from build123d import *

# Parameters (mm, degrees)
SKETCH1_W                  = 170
SKETCH1_H                  = 20
BOSS_EXTRUDE1_DEPTH        = 130
SKETCH2_R                  = 30
SKETCH2_R_2                = 15
BOSS_EXTRUDE3_DEPTH        = 60
BOSS_EXTRUDE3_DEPTH_BACK   = 6
BOSS_EXTRUDE3_2_DEPTH      = 60
BOSS_EXTRUDE3_2_DEPTH_BACK = 6
SKETCH2_4_W                = 55
SKETCH2_4_H                = 55
BOSS_EXTRUDE4_DEPTH        = 6
BOSS_EXTRUDE4_DEPTH_BACK   = 6
SKETCH2_5_W                = 55
SKETCH2_5_H                = 55
SKETCH2_5_R                = 20
BOSS_EXTRUDE5_DEPTH        = 100
RIB10_REACH                = 192.076
SKETCH3_WALL_W             = 453.9773952
SKETCH3_WALL_H             = 15
SKETCH4_R                  = 13
CUT_EXTRUDE1_DEPTH         = 217.573313222


with BuildPart() as part:
    # Sketch1 → Boss-Extrude1 (new body)
    with BuildSketch(Plane.XY):
        Rectangle(SKETCH1_W, SKETCH1_H)
    extrude(amount=-BOSS_EXTRUDE1_DEPTH)



with BuildPart() as body_2:
    # Sketch2 → Boss-Extrude3 (new, two sides)
    with BuildSketch(Plane(origin=(0, 0, 0), x_dir=(1, 0, 0), z_dir=(0, 1, 0))) as boss_extrude3_sk:
        with Locations(Location((-118, 65, 0), (0, 0, 270))):
            Circle(SKETCH2_R)
        with Locations(Location((-118, 65, 0), (0, 0, 270))):
            Circle(SKETCH2_R_2, mode=Mode.SUBTRACT)
    extrude(amount=BOSS_EXTRUDE3_DEPTH)
    extrude(boss_extrude3_sk.sketch, amount=-BOSS_EXTRUDE3_DEPTH_BACK)


with BuildPart() as body_3:
    # Sketch2 → Boss-Extrude3 2 (new, two sides)
    with BuildSketch(Plane(origin=(0, 0, 0), x_dir=(1, 0, 0), z_dir=(0, 1, 0))) as boss_extrude3_2_sk:
        with Locations(Location((118, 65, 0), (0, 0, 270))):
            Circle(SKETCH2_R)
        with Locations(Location((118, 65, 0), (0, 0, 270))):
            Circle(SKETCH2_R_2, mode=Mode.SUBTRACT)
    extrude(amount=BOSS_EXTRUDE3_2_DEPTH)
    extrude(boss_extrude3_2_sk.sketch, amount=-BOSS_EXTRUDE3_2_DEPTH_BACK)


with BuildPart() as part_1:
    add(part.part)

    add(body_2.part)  # Boss-Extrude4 merges body 2

    add(body_3.part)  # Boss-Extrude4 merges body 3
    # Sketch2_4 → Boss-Extrude4 (add, two sides)
    with BuildSketch(Plane(origin=(0, 0, 0), x_dir=(1, 0, 0), z_dir=(0, 1, 0))) as boss_extrude4_sk:
        with BuildLine():
            Line((85, 130), (-85, 130))
            Line((-85, 130), (-85, 110))
            ThreePointArc((-85, 110), (-89.393398282, 99.393398282), (-100, 95))
            Line((-100, 95), (-118, 95))
            ThreePointArc((-118, 95), (-96.786796564, 86.213203436), (-88, 65))
            ThreePointArc((-88, 65), (-96.786796564, 43.786796564), (-118, 35))
            Line((-118, 35), (-100, 35))
            ThreePointArc((-100, 35), (-89.393398282, 30.606601718), (-85, 20))
            Line((-85, 20), (-85, 0))
            Line((-85, 0), (85, 0))
            Line((85, 0), (85, 20))
            ThreePointArc((85, 20), (89.393398282, 30.606601718), (100, 35))
            Line((100, 35), (118, 35))
            ThreePointArc((118, 35), (88, 65), (118, 95))
            Line((118, 95), (100, 95))
            ThreePointArc((100, 95), (89.393398282, 99.393398282), (85, 110))
            Line((85, 110), (85, 130))
        make_face()
        with Locations((0, 65)):
            Rectangle(SKETCH2_4_W, SKETCH2_4_H, mode=Mode.SUBTRACT)
    extrude(amount=BOSS_EXTRUDE4_DEPTH)
    extrude(boss_extrude4_sk.sketch, amount=-BOSS_EXTRUDE4_DEPTH_BACK)

    # Sketch2_5 → Boss-Extrude5 (add)
    with BuildSketch(Plane(origin=(0, 0, 0), x_dir=(1, 0, 0), z_dir=(0, 1, 0))):
        with Locations((0, 65)):
            Rectangle(SKETCH2_5_W, SKETCH2_5_H)
        with Locations(Location((0, 65, 0), (0, 0, 270))):
            Circle(SKETCH2_5_R, mode=Mode.SUBTRACT)
    extrude(amount=BOSS_EXTRUDE5_DEPTH)

    # Sketch3 wall → Rib10 (add, up to next)
    with BuildSketch(Plane(origin=(-58.860010645, 77.5, -65), x_dir=(-0.873236351537, -0.487296905752, 0), z_dir=(0.487296905752, -0.873236351537, 0)), mode=Mode.PRIVATE) as rib10_sk1:
        Rectangle(SKETCH3_WALL_W, SKETCH3_WALL_H)
    rib10_tool1 = extrude(rib10_sk1.sketch, amount=RIB10_REACH, mode=Mode.PRIVATE) - part_1.part
    rib10 = rib10_tool1.solids().sort_by_distance((-58.860010645, 77.5, -65))[0]
    add(rib10)

    # Mirror1: Rib10 across plane
    add(rib10.mirror(Plane(origin=(0, 0, 0), x_dir=(0, 0, 1), z_dir=(1, 0, 0))))

    # Sketch4 → Cut-Extrude1 (cut, through all)
    with BuildSketch(Plane(origin=(0, 10, 0), x_dir=(1, 0, 0), z_dir=(0, 1, 0))):
        with Locations(Location((-63, 108, 0), (0, 0, 270))):
            Circle(SKETCH4_R)
        with Locations(Location((63, 108, 0), (0, 0, 270))):
            Circle(SKETCH4_R)
        with Locations(Location((-63, 22, 0), (0, 0, 270))):
            Circle(SKETCH4_R)
        with Locations(Location((63, 22, 0), (0, 0, 270))):
            Circle(SKETCH4_R)
    extrude(amount=-CUT_EXTRUDE1_DEPTH, mode=Mode.SUBTRACT)


solid = part_1.part
Can you work these out from the model? Positions are in its coordinate system, mm. A direction names the side the tool comes from. Give positions to 0.01 mm unless a question says otherwise; leave off trailing zeros. Loops run counter-clockwise (first coordinate to the right, second up) from the corner with the lowest first, then second, coordinate; pieces in that order, holes last. Notation, with made-up numbers: (63.5, -34.75) - (73.5, -34.75) arc R25 cw to (73.5, -9.75) - close; hole circle Ø1 at (-6, -21.75). An arc over 180 degrees is marked (long way). Answer as a JSON object with one key per item and string values.
Q1. Imagine slicing it at A-A on z = -65. Write out the boundary of the cut face in (x, y).
Geometry says:
{"outline": "(-148, -6) - (-133, -6) - (-133, 60) - (-148, 60) - close; (-103, -6) - (-85, -6) - (-85, -10) - (85, -10) - (85, -6) - (103, -6) - (103, 60) - (90.22, 60) - (27.5, 95) - (27.5, 100) - (20, 100) - (20, 10) - (-20, 10) - (-20, 100) - (-27.5, 100) - (-27.5, 95) - (-90.22, 60) - (-103, 60) - close; (133, -6) - (148, -6) - (148, 60) - (133, 60) - close"}
Q2. Imagine slicing it at B-B on y = 3. Write out the boundary of the cut face in (x, z), plus the area to 3 significant figures.
Geometry says:
{"outline": "(-118, -95) - (-100, -95) arc R15 cw to (-85, -110) - (-85, -130) - (85, -130) - (85, -110) arc R15 cw to (100, -95) - (118, -95) arc R30 ccw to (118, -35) - (100, -35) arc R15 cw to (85, -20) - (85, 0) - (-85, 0) - (-85, -20) arc R15 cw to (-100, -35) - (-118, -35) arc R30 ccw to start; hole circle Ø30 at (-118, -65); hole circle Ø26 at (-63, -108); hole circle Ø26 at (-63, -22); hole circle Ø26 at (63, -108); hole circle Ø26 at (63, -22); hole circle Ø30 at (118, -65)", "area": "25,500 mm²"}
Q3. Imagine slicing it at D-D on x = 0. Write out the boundary of the cut face in (y, z), plus the area to 3 significant figures.
Geometry says:
{"outline": "(-10, -130) - (10, -130) - (10, -92.5) - (100, -92.5) - (100, -85) - (10, -85) - (10, -45) - (100, -45) - (100, -37.5) - (10, -37.5) - (10, 0) - (-10, 0) - close", "area": "3,950 mm²"}
Q4. Will these pins go through, and if not, where does the flat tip stop? P1, Ø19, axis at x = 122.5, z = -59.5, coming from the -Y side; P2, Ø6, axis at x = -105, y = -1, coming from the +Z side; P3, Ø3.5, axis at x = -106, y = -1.5, coming from the -Z side.
Geometry says:
{"P1": "y = -6", "P2": "z = -35", "P3": "z = -95"}
Q5. Imagine slicing it at C-C on y = 54.5. Write out the boundary of the cut face in (x, z), plus the area to 3 significant figures.
Geometry says:
{"outline": "(-88.95, -72.5) - (-27.5, -72.5) - (-27.5, -92.5) - (27.5, -92.5) - (27.5, -72.5) - (88.95, -72.5) arc R30 ccw (long way) to (88.95, -57.5) - (27.5, -57.5) - (27.5, -37.5) - (-27.5, -37.5) - (-27.5, -57.5) - (-88.95, -57.5) arc R30 ccw (long way) to start; hole circle Ø30 at (-118, -65); hole circle Ø40 at (0, -65); hole circle Ø30 at (118, -65)", "area": "7,830 mm²"}
Q6. If I drill on L1, parallel to X at y = 46.5, z = -65; L2, parallel to X at y = 9, z = -65; L3, parallel to Z at x = 64, y = 1, over which ranges is the centre line in solid material (lowest first)?
Geometry says:
{"L1": "-148 to -133, -103 to -20, 20 to 103, 133 to 148", "L2": "-148 to -133, -103 to 103, 133 to 148", "L3": "-130 to -120.96, -95.04 to -34.96, -9.04 to 0"}
Q7. Which directions (+Z, -Z, +X, -X, +Y, -Y) give clear straight access to the entire face, cutting with the end or side of a thin tool? Please do faces 4 (the cylindrical face through (-147.975, 27.462, -66.213)), 5 (the flat face through (109, 0, -95)), 6 (the flat face through (92, 6, -42)), 7 (the flat face through (-92, 6, -89)), 8 (the flat face through (-109, 0, -35)).
Geometry says:
{"face 4": "+Y", "face 5": "-Z, +X, +Y, -Y", "face 6": "+Z, +Y", "face 7": "-Z, +Y", "face 8": "+Z, -X, +Y, -Y"}
Q8. If we mould it in two halves opening along Z, with no side actions, what happens to faces 1 (the flat face through (0, 54, -92.5)), 2 (the cylindrical face through (0.88, 54.37, -84.98)), 3 (the flat face through (85, -7, -64))? For each: pulls with the +Z half, pulls with the -Z half, needs draft (parallel to the pull), parting line crosses it, or undercut.
Geometry says:
{"face 1": "pulls with the -Z half", "face 2": "undercut", "face 3": "needs draft"}
